```python
from build123d import *

# Parameters (mm, degrees)
BOSS_EXTRUDE1_DEPTH = 3
SKETCH3_R           = 1.5
CUT_EXTRUDE1_DEPTH  = 10


with BuildPart() as part:
    # Sketch1 → Boss-Extrude1 (new body)
    with BuildSketch(Plane.XY):
        with BuildLine():
            Line((-3.75, 13.863170633), (-3.75, 23.75))
            ThreePointArc((-3.75, 23.75), (0, 27.5), (3.75, 23.75))
            Line((3.75, 23.75), (3.75, 13.863170633))
            ThreePointArc((3.75, 13.863170633), (4.443854017, 8.640840954), (6.477272727, 3.780864718))
            ThreePointArc((6.477272727, 3.780864718), (0, -7.5), (-6.477272727, 3.780864718))
            ThreePointArc((-6.477272727, 3.780864718), (-4.443854017, 8.640840954), (-3.75, 13.863170633))
        make_face()
        Polygon((0, 3.464101615), (-3, 1.732050808), (-3, -1.732050808), (0, -3.464101615), (3, -1.732050808), (3, 1.732050808), align=None, mode=Mode.SUBTRACT)
    extrude(amount=BOSS_EXTRUDE1_DEPTH)

    # Sketch3 → Cut-Extrude1 (cut)
    with BuildSketch(Plane.XY.offset(3)):
        with Locations((0, 21.5)):
            Circle(SKETCH3_R)
    extrude(amount=-CUT_EXTRUDE1_DEPTH, mode=Mode.SUBTRACT)


solid = part.part
```
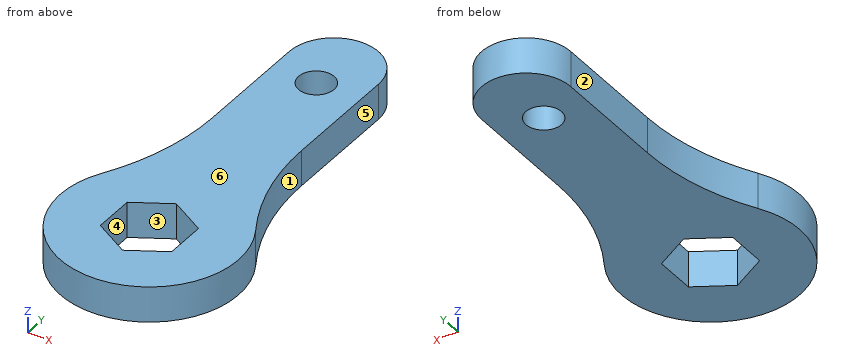
Check sheet for the modelled part. Datum: model origin and axes. Units: mm. Face numbers are marked on the shaded views. A direction names the side the tool comes from. Round coordinates to 2 decimals unless told otherwise and drop trailing zeros. Order: outer loops, then holes, each group sorted by start corner. A loop starts at its lowest first (then second) coordinate and runs counter-clockwise, first axis right, second up. Notation, with made-up numbers: (50, 22) -> (66, 22) arc R17 cw to (66, 42) -> close; hole circle Ø9 at (17.25, -6). An arc over 180 degrees is marked (long way). Use CSV: the item, a comma, the result in double quotes.
(1) Cross-section at C-C (y = 15.5). Record the boundary of the cut face in (x, z), and give its area (3 significant figures).
Worked out:
outline,"(-3.75, 0) -> (3.75, 0) -> (3.75, 3) -> (-3.75, 3) -> close"
area,"22.5 mm²"
(2) Draft check along X on the marked faces 1, 2 and 3. Enter one of: pulls with the +X half, pulls with the -X half, needs draft (parallel to the pull), parting line crosses it, or undercut.
Worked out:
face 1,"pulls with the +X half"
face 2,"pulls with the -X half"
face 3,"undercut"
(3) Cross-section at B-B (x = 2). Record the boundary of the cut face in (y, z).
Worked out:
outline,"(-7.23, 0) -> (-2.31, 0) -> (-2.31, 3) -> (-7.23, 3) -> close; (2.31, 0) -> (26.92, 0) -> (26.92, 3) -> (2.31, 3) -> close"
(4) Material ranges on line 1 along Y through (x, z) = (-0.25, 1.45); line 2 along Y through (x, z) = (1.75, 0.65); line 3 along X through (y, z) = (-1, 1.7), recorded low to high. Write a range as from..to.
Worked out:
line 1,"-7.5..-3.32, 3.32..20.02, 22.98..27.49"
line 2,"-7.29..-2.45, 2.45..27.07"
line 3,"-7.43..-3, 3..7.43"
(5) Depth check by flat-ended pin: pin 1 (1.5 mm diameter, centred on y = 18.5, z = 2, fed in from -X); pin 2 (3.5 mm diameter, centred on x = 0, y = 21.5, fed in from -Z). Enter the tip coordinate at first touch or a pass-through.
Worked out:
pin 1,"x = -3.75"
pin 2,"z = 0"
(6) Cross-section at A-A (y = 21.5). Record the boundary of the cut face in (x, z).
Worked out:
outline,"(-3.75, 0) -> (-1.5, 0) -> (-1.5, 3) -> (-3.75, 3) -> close; (1.5, 0) -> (3.75, 0) -> (3.75, 3) -> (1.5, 3) -> close"
(7) Cross-section at D-D (x = 6). Record the boundary of the cut face in (y, z), and give its area (3 significant figures).
Worked out:
outline,"(-4.5, 0) -> (4.65, 0) -> (4.65, 3) -> (-4.5, 3) -> close"
area,"27.4 mm²"
(8) Tool access check on the marked faces 4, 5 and 6. Record the directions out of +Z, -Z, +X, -X, +Y, -Y that give a thin tool (end or side, any length) a straight path to the whole face; none if there is none.
Worked out:
face 4,"+Z, -Z"
face 5,"+Z, -Z, +X, +Y"
face 6,"+Z, +X, -X, +Y, -Y"
